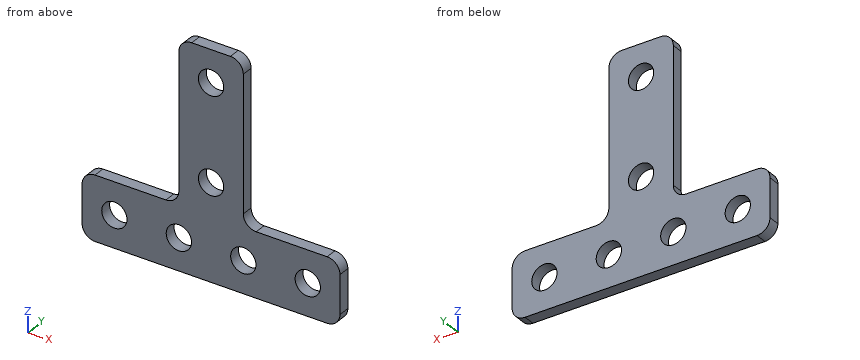
from build123d import *

# Parameters (mm, degrees)
SKETCH1_R           = 2.4892
SKETCH1_W           = 12.7
SKETCH1_H           = 31.75
BOSS_EXTRUDE1_DEPTH = 2.286
FILLET1_R           = 2.54


with BuildPart() as part:
    # Sketch1 → Boss-Extrude1 (new body)
    # profile 1 of 2: a face of its own
    with BuildSketch(Plane(origin=(0, 0, 0), x_dir=(1, 0, 0), z_dir=(0, 1, 0))):
        Polygon((-19.047100434, 31.75), (0, 31.75), (12.7, 31.75), (31.75, 31.75), (31.75, 44.45), (-19.047100434, 44.45), align=None)
        with Locations(Location((-12.697100434, 38.1, 0), (0, 0, 270))):
            Circle(SKETCH1_R, mode=Mode.SUBTRACT)
        with Locations(Location((0.002899566, 38.1, 0), (0, 0, 270))):
            Circle(SKETCH1_R, mode=Mode.SUBTRACT)
        with Locations(Location((12.702899566, 38.1, 0), (0, 0, 270))):
            Circle(SKETCH1_R, mode=Mode.SUBTRACT)
        with Locations(Location((25.4, 38.1, 0), (0, 0, 270))):
            Circle(SKETCH1_R, mode=Mode.SUBTRACT)
    # profile 2 of 2: a face of its own
    with BuildSketch(Plane(origin=(0, 0, 0), x_dir=(1, 0, 0), z_dir=(0, 1, 0))):
        with Locations((6.35, 15.875)):
            Rectangle(SKETCH1_W, SKETCH1_H)
        with Locations(Location((6.35, 25.4, 0), (0, 0, 270))):
            Circle(SKETCH1_R, mode=Mode.SUBTRACT)
        with Locations(Location((6.35, 6.35, 0), (0, 0, 270))):
            Circle(SKETCH1_R, mode=Mode.SUBTRACT)
    extrude(amount=BOSS_EXTRUDE1_DEPTH)

    # Fillet1
    fillet1_edges = [part.edges().sort_by_distance(p)[0] for p in [
        (-19.047100434, 1.143, -31.75),
        (-19.047100434, 1.143, -44.45),
        (31.75, 1.143, -44.45),
        (31.75, 1.143, -31.75),
        (12.7, 1.143, -31.75),
        (12.7, 1.143, 0),
        (0, 1.143, 0),
        (0, 1.143, -31.75),
    ]]
    fillet(fillet1_edges, radius=FILLET1_R)


solid = part.part
Geometry: final body of the model. Coordinates: model frame, mm. Give positions to 0.01 mm unless a question says otherwise; leave off trailing zeros. Loops run counter-clockwise (first coordinate to the right, second up) from the corner with the lowest first, then second, coordinate; pieces in that order, holes last. Notation, with made-up numbers: (30.25, 86.5) - (83.25, 86.5) arc R29 ccw to (83.25, 112.5) - close; hole circle Ø10 at (18, -31.75). An arc over 180 degrees is marked (long way). One line per question, with ' | ' between items. Start each with the question number.
(1) Ray query, line 1 (X direction, y = 1.6, z = -38.1); line 2 (X direction, y = 1.6, z = -6.35); line 3 (Z direction, x = 4.5, y = 1.5). Return the intervals inside material, ascending. Write a range as from..to.
(2) Section query D-D on x = 6.35. Return loops of the section in (y, z), then the cut area to 3 significant figures.
(3) Contact query for a flat-ended pin moving along its axis: pin 1 (4.5 mm diameter, centred on x = 25.4, z = -38.1, fed in from +Y). Output: stop coordinate, or through.
(4) Section query C-C on y = 1.65. Return loops of the section in (x, z).
(5) Section query A-A on z = -6.35. Return loops of the section in (x, y).
(6) Section query B-B on x = 25.4. Return loops of the section in (y, z).
The answers:
1) line 1: -19.05..-15.19, -10.21..-2.49, 2.49..10.21, 15.19..22.91, 27.89..31.75 | line 2: 0..3.86, 8.84..12.7 | line 3: -44.45..-27.07, -23.73..-8.02, -4.68..0
2) outline: (0, -44.45) - (2.29, -44.45) - (2.29, -27.89) - (0, -27.89) - close; (0, -22.91) - (2.29, -22.91) - (2.29, -8.84) - (0, -8.84) - close; (0, -3.86) - (2.29, -3.86) - (2.29, 0) - (0, 0) - close | area: 78.9 mm2
3) pin 1: through
4) outline: (-19.05, -41.91) arc R2.54 ccw to (-16.51, -44.45) - (29.21, -44.45) arc R2.54 ccw to (31.75, -41.91) - (31.75, -34.29) arc R2.54 ccw to (29.21, -31.75) - (15.24, -31.75) arc R2.54 cw to (12.7, -29.21) - (12.7, -2.54) arc R2.54 ccw to (10.16, 0) - (2.54, 0) arc R2.54 ccw to (0, -2.54) - (0, -29.21) arc R2.54 cw to (-2.54, -31.75) - (-16.51, -31.75) arc R2.54 ccw to (-19.05, -34.29) - close; hole circle Ø4.98 at (-12.7, -38.1); hole circle Ø4.98 at (0, -38.1); hole circle Ø4.98 at (6.35, -25.4); hole circle Ø4.98 at (6.35, -6.35); hole circle Ø4.98 at (12.7, -38.1); hole circle Ø4.98 at (25.4, -38.1)
5) outline: (0, 0) - (3.86, 0) - (3.86, 2.29) - (0, 2.29) - close; (8.84, 0) - (12.7, 0) - (12.7, 2.29) - (8.84, 2.29) - close
6) outline: (0, -44.45) - (2.29, -44.45) - (2.29, -40.59) - (0, -40.59) - close; (0, -35.61) - (2.29, -35.61) - (2.29, -31.75) - (0, -31.75) - close
